Read the model definition and answer for the solid it produces. Units are mm, in the model's axes. Face numbers are marked on the shaded views. Coordinates: 2 decimals unless noted, no trailing zeros. Write each loop counter-clockwise with the first axis right and the second up, starting at its lowest first coordinate (ties: lowest second). Pieces come first, ordered by that corner, then holes. Notation, with made-up numbers: (46.5, 53) -> (99.5, 53) arc R26 ccw to (99.5, 74) -> close; hole circle Ø4 at (7.5, 23). An arc over 180 degrees is marked (long way). Use CSV: the item, a comma, the result in double quotes.
from build123d import *

# Parameters (mm, degrees)
F0_R     = 63.5
F0_R_2   = 60
F1_DEPTH = 260
F2_R     = 63.806252
F3_DEPTH = 3
F4_R     = 63.968913
F5_DEPTH = 3


with BuildPart() as f1:
    # F0 (on Top) → F1 (new body)
    with BuildSketch(Plane.XY):
        Circle(F0_R)
        Circle(F0_R_2, mode=Mode.SUBTRACT)
    extrude(amount=F1_DEPTH)

    # F2 (on face) → F3 (join)
    with BuildSketch(Plane(origin=(0, 0, 0), x_dir=(1, 0, 0), z_dir=(0, 0, -1))):
        Circle(F2_R)
    extrude(amount=F3_DEPTH)

    # F4 (on face) → F5 (join)
    with BuildSketch(Plane.XY.offset(260)):
        Circle(F4_R)
    extrude(amount=F5_DEPTH)


solid = f1.part
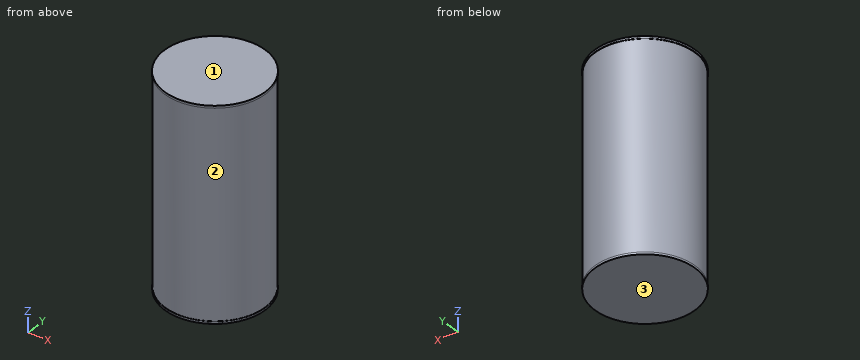
1. A cutting plane is placed at C-C (z = 136). Give the vertices of the cut face in (x, y), and give its area (3 significant figures).
Solutions:
outline,"circle Ø127 at (0, 0); hole circle Ø120 at (0, 0)"
area,"1,360 mm^2"
2. Each of these flat-tipped pins is pushed along its axis until it touches: pin 1 Ø6 at (x, z) = (36, 116) entering from -Y; pin 2 Ø12 at (y, z) = (-0.5, 61) entering from +X; pin 3 Ø3 at (y, z) = (-23.5, 160.5) entering from +X. Where does it stop, or does it pass through?
Solutions:
pin 1,"stops at y = -54.25"
pin 2,"stops at x = 63.5"
pin 3,"stops at x = 59.57"
3. For a pull along Z with two mould halves and no side action, classify the marked faces 1, 2 and 3 as pulls with the +Z half, pulls with the -Z half, needs draft (parallel to the pull), parting line crosses it, or undercut.
Solutions:
face 1,"pulls with the +Z half"
face 2,"undercut"
face 3,"pulls with the -Z half"
4. Find the intervals of material crossed by line 1 along Z through (x, y) = (-1.5, -41); line 2 along Y through (x, z) = (0, 159.5); line 3 along Y through (x, z) = (42, 170), in increasing order.
Solutions:
line 1,"z = -3 to 0, 260 to 263"
line 2,"y = -63.5 to -60, 60 to 63.5"
line 3,"y = -47.63 to -42.85, 42.85 to 47.63"
5. A cutting plane is placed at A-A (x = 0). Give the vertices of the cut face in (y, z).
Solutions:
outline,"(-63.97, 260) -> (-63.5, 260) -> (-63.5, 0) -> (-63.81, 0) -> (-63.81, -3) -> (63.81, -3) -> (63.81, 0) -> (63.5, 0) -> (63.5, 260) -> (63.97, 260) -> (63.97, 263) -> (-63.97, 263) -> close; hole (-60, 0) -> (60, 0) -> (60, 260) -> (-60, 260) -> close"
